Can you work these out from the model? Positions are in its coordinate system, mm. A direction names the side the tool comes from. Coordinates: 2 decimals unless noted, no trailing zeros. Order: outer loops, then holes, each group sorted by start corner. A loop starts at its lowest first (then second) coordinate and runs counter-clockwise, first axis right, second up. Notation, with made-up numbers: (82, 10.25) - (129, 10.25) arc R24 ccw to (129, 37.25) - close; hole circle Ø9 at (-39.5, 28). An arc over 180 degrees is marked (long way). Return JSON: item names as keys, results as strings. Group by question number.
1) For pin 1 Ø1.2 at (x, z) = (30.5, 2.5) entering from -Y; pin 2 Ø10 at (x, y) = (8.5, 3.5) entering from -Z; pin 3 Ø2 at (y, z) = (-18.5, 2) entering from -X; pin 4 Ø2 at (y, z) = (-15, 2) entering from +X, each with a flat end and sliding along its axis, tell me the tip position at first contact or that it passes through.
2) If we mould it in two halves opening along Y, with no side actions, what happens to faces 4 (the face through (17, -12.4, 2)), 5 (the face through (-26.95, -1.4, 1.97)), 6 (the face through (-20.18, 2.87, 1.97))? For each: pulls with the +Y half, pulls with the -Y half, needs draft (parallel to the pull), parting line crosses it, or undercut.
3) Imagine slicing it at D-D (y = -9). Write out the boundary of the cut face in (x, z), and give its area (3 significant figures).
4) If I drill on line 1 along Y through (x, z) = (45.5, 0.9); line 2 along Y through (x, z) = (24, 0.6); line 3 along X through (y, z) = (-8.5, 3.05), over which ranges is the centre line in solid material (lowest first)?
5) Imagine slicing it at C-C (x = 16). Write out the boundary of the cut face in (y, z).
6) Which directions (+Z, -Z, +X, -X, +Y, -Y) give clear straight access to the entire face, cutting with the end or side of a thin tool? Please do faces 1 (the face through (18, -2.4, 2)), 2 (the face through (8, -8, 0)), 3 (the face through (-26.86, -12.95, 1.97)).
7) Imagine slicing it at A-A (z = 2.5). Write out the boundary of the cut face in (x, y).
8) Imagine slicing it at B-B (y = -5.5). Write out the boundary of the cut face in (x, z), and give its area (3 significant figures).
```python
from build123d import *

# Parameters (mm, degrees)
ESBO_O1_R                = 2.55
RESSALTO_EXTRUS_O1_DEPTH = 4


with BuildPart() as part:
    # Esboço1 → Ressalto-extrusão1 (new body)
    with BuildSketch(Plane.XY):
        Polygon((52.704190952, -2.400470185), (-17.136160755, -2.400470185), (-23.307642689, 8.288850082), (-30.235845919, 4.288850082), (-23.57078241, -7.255378552), (-30.235845919, -18.799607186), (-23.301725869, -22.803023264), (-17.295809048, -12.400470185), (52.704190952, -12.400470185), align=None)
        with Locations((45.538806525, -7.255378552)):
            Circle(ESBO_O1_R, mode=Mode.SUBTRACT)
    extrude(amount=RESSALTO_EXTRUS_O1_DEPTH)


solid = part.part
```
Calculated:
{
 "1": {"pin 1": "y = -12.4", "pin 2": "through", "pin 3": "x = -30.24", "pin 4": "x = -18.22"},
 "2": {"face 4": "pulls with the -Y half", "face 5": "undercut", "face 6": "pulls with the +Y half"},
 "3": {"outline": "(-24.58, 0) - (43.68, 0) - (43.68, 4) - (-24.58, 4) - close; (47.4, 0) - (52.7, 0) - (52.7, 4) - (47.4, 4) - close", "area": "294 mm2"},
 "4": {"line 1": "-12.4 to -9.81, -4.71 to -2.4", "line 2": "-12.4 to -2.4", "line 3": "-24.29 to 43.31, 47.76 to 52.7"},
 "5": {"outline": "(-12.4, 0) - (-2.4, 0) - (-2.4, 4) - (-12.4, 4) - close"},
 "6": {"face 1": "+Z, -Z, +X, +Y", "face 2": "-Z, +X, -X, +Y, -Y", "face 3": "+Z, -Z, -X"},
 "7": {"outline": "(-30.24, -18.8) - (-23.3, -22.8) - (-17.3, -12.4) - (52.7, -12.4) - (52.7, -2.4) - (-17.14, -2.4) - (-23.31, 8.29) - (-30.24, 4.29) - (-23.57, -7.26) - close; hole circle Ø5.1 at (45.54, -7.26)"},
 "8": {"outline": "(-24.58, 0) - (43.69, 0) - (43.69, 4) - (-24.58, 4) - close; (47.39, 0) - (52.7, 0) - (52.7, 4) - (47.39, 4) - close", "area": "294 mm2"}
}
